from build123d import *

# Parameters (mm, degrees)
F0_W     = 10
F0_H     = 76.8
F0_H_2   = 10
F0_W_2   = 100
F0_H_3   = 113.2
F1_DEPTH = 100
F3_DEPTH = 5
F4_R     = 2
F6_D     = 8.5


with BuildPart() as f1:
    # F0 (on Front) → F1 (new body, symmetric)
    with BuildSketch(Plane.XZ):
        with Locations((-22.584166, 61.6)):
            Rectangle(F0_W, F0_H)
        with Locations((-22.584166, 18.2)):
            Rectangle(F0_W, F0_H_2)
        with Locations((32.415834, 18.2)):
            Rectangle(F0_W_2, F0_H_2)
        with Locations((-22.584166, -43.4)):
            Rectangle(F0_W, F0_H_3)
    extrude(amount=F1_DEPTH, both=True)

    # F2 (on Front) → F3 (join, symmetric)
    with BuildSketch(Plane.XZ):
        Polygon((-17.584166, 13.2), (-17.584166, -56.8), (52.415834, 13.2), align=None)
    extrude(amount=F3_DEPTH, both=True)

    # F4
    f4_edges = [f1.edges().sort_by_distance(p)[0] for p in [
        (17.415834, -5, 13.2),
        (-17.584166, -5, -21.8),
        (-17.584166, -52.5, 13.2),
        (-17.584166, 52.5, 13.2),
        (-17.584166, 5, -21.8),
        (17.415834, 5, 13.2),
    ]]
    fillet(f4_edges, radius=F4_R)

    # F6 (through all)
    with Locations(Plane.YZ.offset(-17.584166)):
        with Locations((-85, 85), (85, 85), (85, -85), (-85, -85)):
            Hole(F6_D / 2)


solid = f1.part
The model under review builds one solid part; all positions refer to its coordinate system, in mm. A direction names the side the tool comes from. Coordinates: 2 decimals unless noted, no trailing zeros. Write each loop counter-clockwise with the first axis right and the second up, starting at its lowest first coordinate (ties: lowest second). Pieces come first, ordered by that corner, then holes. Notation, with made-up numbers: (81, 80.25) -> (106, 80.25) arc R3 cw to (106, 84.25) -> close; hole circle Ø1 at (55, 75.5). An arc over 180 degrees is marked (long way). Answer in a Markdown table with one row per item.
1. Draft analysis for pull direction Z (two halves, no side actions). For faces 5 (the flat face through (-23, -1, -100)), 6 (the cylindrical face through (-22.65, 85.92, -89.15)), 7 (the flat face through (32, -1, 23.2)), 8 (the cylindrical face through (-22.65, -84.08, 80.85)), state which applies: +Z half, -Z half, draft (parallel to the pull), parting line (faces both ways), or undercut.
Answers below:
| item | result |
|---|---|
| face 5 | -Z half |
| face 6 | undercut |
| face 7 | +Z half |
| face 8 | undercut |
2. We need section B-B, the plane z = 85. State the section outline as (x, y) points.
Answers below:
| item | result |
|---|---|
| outline | (-27.58, -100) -> (-17.58, -100) -> (-17.58, -89.25) -> (-27.58, -89.25) -> close; (-27.58, -80.75) -> (-17.58, -80.75) -> (-17.58, 80.75) -> (-27.58, 80.75) -> close; (-27.58, 89.25) -> (-17.58, 89.25) -> (-17.58, 100) -> (-27.58, 100) -> close |
3. Wall thickness on probe 1 along Z at (x, y) = (-23, -85); probe 2 along Z at (x, y) = (72.5, -86); probe 3 along X at (y, z) = (-23.5, -35.5): over which ranges is each line inside the solid? List them lowest first. Write a range as [from, to].
Answers below:
| item | result |
|---|---|
| probe 1 | z = [-100, -89.25], [-80.75, 80.75], [89.25, 100] |
| probe 2 | z = [13.2, 23.2] |
| probe 3 | x = [-27.58, -17.58] |
4. We need section C-C, the plane y = -67. State the section outline as (x, z) points, and give its area (3 significant figures).
Answers below:
| item | result |
|---|---|
| outline | (-27.58, -100) -> (-17.58, -100) -> (-17.58, 11.2) arc R2 cw to (-15.58, 13.2) -> (82.42, 13.2) -> (82.42, 23.2) -> (-17.58, 23.2) -> (-17.58, 100) -> (-27.58, 100) -> close |
| area | 3,000 mm^2 |
5. Clearance check with a flat-ended pin moving along its axis: pin 1 Ø12 at (y, z) = (73, -74.5) entering from +X. State where the tip first meets the part, or that it passes through.
Answers below:
| item | result |
|---|---|
| pin 1 | stops at x = -17.58 |
6. For faces 1 (the flat face through (-17.584, -1, 61)), 2 (the flat face through (10, 5, -14)), 3 (the flat face through (10, -5, -14)), 4 (the flat face through (55, -1, 13.2)), list the 3-axis set-ups (+Z, -Z, +X, -X, +Y, -Y) from which the entire face can be reached by the end or side of a thin tool; tool diameter is ignored.
Answers below:
| item | result |
|---|---|
| face 1 | +Z, +X, +Y, -Y |
| face 2 | -Z, +X, +Y |
| face 3 | -Z, +X, -Y |
| face 4 | -Z, +X |
7. We need section A-A, the plane y = 85. State the section outline as (x, z) points.
Answers below:
| item | result |
|---|---|
| outline | (-27.58, -100) -> (-17.58, -100) -> (-17.58, -89.25) -> (-27.58, -89.25) -> close; (-27.58, -80.75) -> (-17.58, -80.75) -> (-17.58, 11.2) arc R2 cw to (-15.58, 13.2) -> (82.42, 13.2) -> (82.42, 23.2) -> (-17.58, 23.2) -> (-17.58, 80.75) -> (-27.58, 80.75) -> close; (-27.58, 89.25) -> (-17.58, 89.25) -> (-17.58, 100) -> (-27.58, 100) -> close |
8. We need section D-D, the plane x = 75. State the section outline as (y, z) points, and give its area (3 significant figures).
Answers below:
| item | result |
|---|---|
| outline | (-100, 13.2) -> (100, 13.2) -> (100, 23.2) -> (-100, 23.2) -> close |
| area | 2,000 mm^2 |
